For this review, take the finished solid that the model builds, in its own axes (mm). Face numbers are marked on the shaded views. A direction names the side the tool comes from. Coordinates: 2 decimals unless noted, no trailing zeros. Write each loop counter-clockwise with the first axis right and the second up, starting at its lowest first coordinate (ties: lowest second). Pieces come first, ordered by that corner, then holes. Notation, with made-up numbers: M 62,16 L 91,16 A14 ccw 91,31 Z; hole C -20,75 d4. An arc over 180 degrees is marked long. Return JSON: item names as keys, results as strings.
```python
from build123d import *

# Parameters (mm, degrees)
CROQUIS1_W              = 21.8
CROQUIS1_H              = 50
SALIENTE_EXTRUIR1_DEPTH = 21.8
CROQUIS6_R              = 2
CORTAR_EXTRUIR2_DEPTH   = 21.8
CORTAR_EXTRUIR4_REACH   = 60.741
CROQUIS11_R             = 3.5
CROQUIS11_W             = 3.4
CROQUIS11_H             = 8.4
REDONDEO1_R             = 5
CROQUIS13_R             = 3.5
CORTAR_EXTRUIR6_DEPTH   = 3.5
CROQUIS15_W             = 3.4
CROQUIS15_H             = 8.4
SALIENTE_EXTRUIR2_DEPTH = 13


with BuildPart() as part:
    # Croquis1 → Saliente-Extruir1 (new body)
    with BuildSketch(Plane(origin=(0, 0, 0), x_dir=(0, 0, -1), z_dir=(1, 0, 0))):
        with Locations((-10.9, -25)):
            Rectangle(CROQUIS1_W, CROQUIS1_H)
    extrude(amount=SALIENTE_EXTRUIR1_DEPTH)

    # Croquis6 → Cortar-Extruir2 (cut)
    with BuildSketch(Plane.ZY):
        with Locations((10.9, -22)):
            Circle(CROQUIS6_R)
        with Locations((10.9, -7)):
            Circle(CROQUIS6_R)
    extrude(amount=-CORTAR_EXTRUIR2_DEPTH, mode=Mode.SUBTRACT)

    # Croquis11 → Cortar-Extruir4 (cut, up to next)
    with BuildSketch(Plane.XZ.offset(50), mode=Mode.PRIVATE) as cortar_extruir4_sk1:
        with Locations(Location((13.4, 10.9, 0), (0, 0, 270))):
            Circle(CROQUIS11_R)
    cortar_extruir4_tool1 = extrude(cortar_extruir4_sk1.sketch, amount=-CORTAR_EXTRUIR4_REACH, mode=Mode.PRIVATE) & part.part
    # Croquis11 → Cortar-Extruir4 (cut, up to next)
    with BuildSketch(Plane.XZ.offset(50), mode=Mode.PRIVATE) as cortar_extruir4_sk2:
        with Locations((7.2, 10.9)):
            Rectangle(CROQUIS11_W, CROQUIS11_H)
    cortar_extruir4_tool2 = extrude(cortar_extruir4_sk2.sketch, amount=-CORTAR_EXTRUIR4_REACH, mode=Mode.PRIVATE) & part.part
    add(cortar_extruir4_tool1.solids().sort_by_distance((13.4, -50, 10.9))[0], mode=Mode.SUBTRACT)
    add(cortar_extruir4_tool2.solids().sort_by_distance((7.2, -50, 10.9))[0], mode=Mode.SUBTRACT)

    # Redondeo1
    # the kernel refuses this fillet: 5 mm, written as the material it takes off along each edge
    with BuildSketch(Plane(origin=(21.8, -50, 34.3), x_dir=(0, 1, 0), z_dir=(0, 0, -1)), Plane(origin=(0, 0, -12.5), x_dir=(1, 0, 0), z_dir=(0, 0, 1))) as redondeo1_piece_1:
        with BuildLine():
            CenterArc((REDONDEO1_R, -REDONDEO1_R), REDONDEO1_R, 90, 90)
            Line((0, -REDONDEO1_R), (0, 0))
            Line((0, 0), (REDONDEO1_R, 0))
        make_face()
    extrude(amount=46.8, mode=Mode.SUBTRACT)
    with BuildSketch(Plane(origin=(21.8, 0, -12.5), x_dir=(-1, 0, 0), z_dir=(0, 0, 1)), Plane(origin=(0, -50, 34.3), x_dir=(0, 1, 0), z_dir=(0, 0, -1))) as redondeo1_piece_2:
        with BuildLine():
            CenterArc((REDONDEO1_R, REDONDEO1_R), REDONDEO1_R, 180, 90)
            Line((0, REDONDEO1_R), (0, 0))
            Line((0, 0), (REDONDEO1_R, 0))
        make_face()
    extrude(amount=46.8, mode=Mode.SUBTRACT)

    # Croquis13 → Cortar-Extruir6 (cut)
    with BuildSketch(Plane.ZY):
        with Locations((10.9, -7)):
            Circle(CROQUIS13_R)
        with Locations((10.9, -22)):
            Circle(CROQUIS13_R)
    extrude(amount=-CORTAR_EXTRUIR6_DEPTH, mode=Mode.SUBTRACT)

    # Croquis15 → Saliente-Extruir2 (add)
    with BuildSketch(Plane.XZ.offset(50)):
        with Locations((7.2, 10.9)):
            Rectangle(CROQUIS15_W, CROQUIS15_H)
        with BuildLine():
            ThreePointArc((16.8, 10.069337614), (16.9, 10.9), (16.8, 11.730662386))
            ThreePointArc((16.8, 11.730662386), (9.9, 10.9), (16.8, 10.069337614))
        make_face()
    extrude(amount=-SALIENTE_EXTRUIR2_DEPTH)


solid = part.part
```
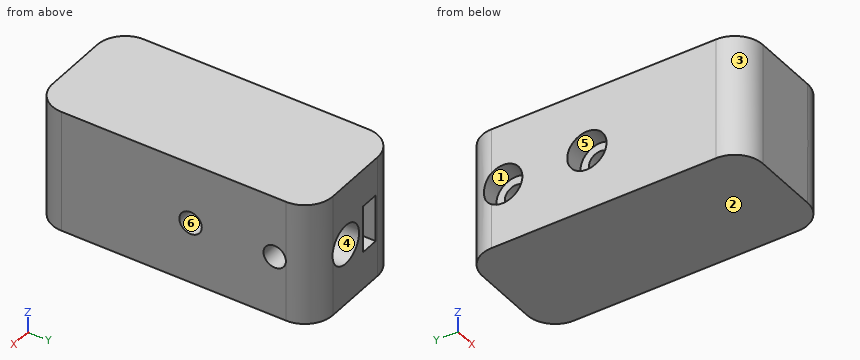
1. Draft analysis for pull direction Y (two halves, no side actions). For the marked faces 1, 2 and 3, state which applies: +Y half, -Y half, draft (parallel to the pull), parting line (faces both ways), or undercut.
Checks:
{"face 1": "undercut", "face 2": "draft", "face 3": "-Y half"}
2. We need section C-C (y = -33.5). State the section outline as (x, z) points, plus the area to 3 significant figures.
Checks:
{"outline": "M 0,0 L 21.8,0 L 21.8,21.8 L 0,21.8 Z; hole M 5.5,6.7 L 8.9,6.7 L 8.9,15.1 L 5.5,15.1 Z; hole C 13.4,10.9 d7", "area": "408 mm2"}
3. For the marked faces 4, 5 and 6, list the 3-axis set-ups (+Z, -Z, +X, -X, +Y, -Y) from which the entire face can be reached by the end or side of a thin tool; tool diameter is ignored.
Checks:
{"face 4": "+Y", "face 5": "-X", "face 6": "+X, -X"}
4. Clearance check with a flat-ended pin moving along its axis: pin 1 Ø3.5 at (y, z) = (-6.5, 10) entering from -X. State where the tip first meets the part, or that it passes through.
Checks:
{"pin 1": "x = 3.5"}
5. Wall thickness on L1, parallel to Z at x = 1.9, y = -7; L2, parallel to Z at x = 8.75, y = -20; L3, parallel to X at y = -33.5, z = 9: over which ranges is each line inside the solid? List them lowest first. Write a range as from..to.
Checks:
{"L1": "0..7.4, 14.4..21.8", "L2": "0..6.7, 15.1..21.8", "L3": "0..5.5, 8.9..10.46, 16.34..21.8"}
6. We need section D-D (x = 6.5). State the section outline as (y, z) points.
Checks:
{"outline": "M -50,0 L 0,0 L 0,6.7 L -37,6.7 L -37,15.1 L 0,15.1 L 0,21.8 L -50,21.8 Z"}
7. We need section A-A (y = -22). State the section outline as (x, z) points.
Checks:
{"outline": "M 0,0 L 21.8,0 L 21.8,8.9 L 16.27,8.9 A3.5 cw 10.53,8.9 L 8.9,8.9 L 8.9,6.7 L 5.5,6.7 L 5.5,8.9 L 3.5,8.9 L 3.5,7.4 L 0,7.4 Z; M 0,14.4 L 3.5,14.4 L 3.5,12.9 L 5.5,12.9 L 5.5,15.1 L 8.9,15.1 L 8.9,12.9 L 10.53,12.9 A3.5 cw 16.27,12.9 L 21.8,12.9 L 21.8,21.8 L 0,21.8 Z"}
8. We need section B-B (z = 19.25). State the section outline as (x, y) points.
Checks:
{"outline": "M 0,-45 A5 ccw 5,-50 L 16.8,-50 A5 ccw 21.8,-45 L 21.8,-5 A5 ccw 16.8,0 L 5,0 A5 ccw 0,-5 Z"}
